```python
from build123d import *

# Parameters (mm, degrees)
SKETCH1_W           = 10
SKETCH1_H           = 10
BOSS_EXTRUDE1_DEPTH = 50
BOSS_EXTRUDE2_START = -45
SKETCH2_R           = 20
BOSS_EXTRUDE2_DEPTH = 2.5
FILLET2_R           = 2
FILLET3_R           = 5
FILLET4_R           = 5
SCALE1_SCALE        = 1.5


with BuildPart() as part:
    # Sketch1 → Boss-Extrude1 (new, symmetric)
    with BuildSketch(Plane(origin=(0, 0, 0), x_dir=(1, 0, 0), z_dir=(0, 1, 0))):
        Rectangle(SKETCH1_W, SKETCH1_H)
    extrude(amount=BOSS_EXTRUDE1_DEPTH, both=True)

    # Sketch2 → Boss-Extrude2 (add, symmetric)
    with BuildSketch(Plane(origin=(0, 50, 0), x_dir=(1, 0, 0), z_dir=(0, 1, 0)).offset(BOSS_EXTRUDE2_START)):
        with Locations(Location((0, 0, 0), (0, 0, 270))):
            Circle(SKETCH2_R)
    extrude(amount=BOSS_EXTRUDE2_DEPTH, both=True)

    # Fillet2
    fillet2_edges = [part.edges().sort_by_distance(p)[0] for p in [
        (5, -23.75, 5),
        (-5, -23.75, 5),
        (-5, -23.75, -5),
        (5, -23.75, -5),
    ]]
    fillet(fillet2_edges, radius=FILLET2_R)

    # Fillet3
    fillet3_edges = [part.edges().sort_by_distance(p)[0] for p in [
        (-5, 28.75, -5),
        (-5, 28.75, 5),
        (5, 28.75, 5),
        (5, 28.75, -5),
    ]]
    fillet(fillet3_edges, radius=FILLET3_R - 0.0001)  # a hair under: the kernel refuses the full size

    # Fillet4
    fillet4_edges = [part.edges().sort_by_distance(p)[0] for p in [
        (3.535563195, 50, -3.535563195),
        (3.535563195, 50, 3.535563195),
        (-3.535563195, 50, 3.535563195),
        (-3.535563195, 50, -3.535563195),
    ]]
    fillet(fillet4_edges, radius=FILLET4_R - 0.0001)  # a hair under: the kernel refuses the full size


with BuildPart() as part_1:
    # Scale1: scaled about (0, 0.040894901, 0)
    add(part.part.scale(SCALE1_SCALE).moved(Location((0, -0.02044745, 0))))


solid = part_1.part
```
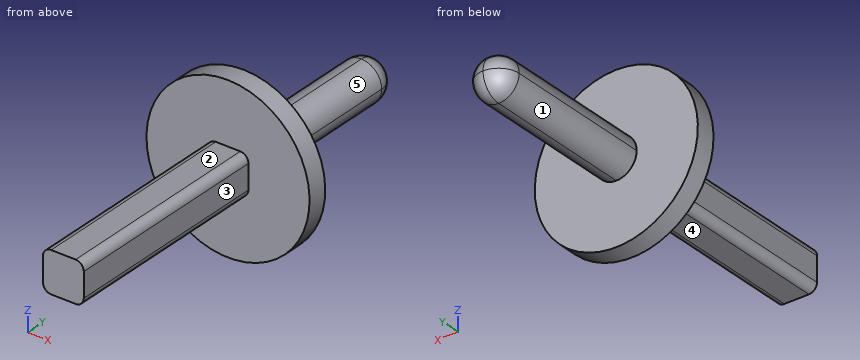
Geometry check sheet. Reference: the model listing, model coordinates, mm. Face numbers are marked on the shaded views. A direction names the side the tool comes from. Round coordinates to 2 decimals unless told otherwise and drop trailing zeros. Order: outer loops, then holes, each group sorted by start corner. A loop starts at its lowest first (then second) coordinate and runs counter-clockwise, first axis right, second up. Notation, with made-up numbers: M 5.25,-1.75 L 33.25,-1.75 A24 ccw 33.25,29.25 Z; hole C 69.25,-22.5 d8. An arc over 180 degrees is marked long. Write item = value, one per line.
Q1. Depth check by flat-ended pin: pin 1 Ø6 at (x, z) = (-16.5, -21.5) entering from -Y; pin 2 Ø10 at (y, z) = (-24, 2) entering from -X; pin 3 Ø7 at (x, y) = (1.5, -31) entering from +Z; pin 4 Ø1 at (y, z) = (-31, 9) entering from -X. Enter the tip coordinate at first touch or a pass-through.
Answer block:
pin_1 = 3.73
pin_2 = -7.5
pin_3 = 7.5
pin_4 = through
Q2. Scan lines: line 1 (Y direction, x = 14.5, z = -25); line 2 (Y direction, x = -4.5, z = -6.5); line 3 (Z direction, x = 19, y = 10). Record each from-to range of solid material in increasing order.
Answer block:
line_1 = 3.73 to 11.23
line_2 = -75.02 to 11.23
line_3 = -23.22 to 23.22
Q3. Section check D-D (x = 9). Enter the section's corners in (y, z).
Answer block:
outline = M 3.73,-28.62 L 11.23,-28.62 L 11.23,28.62 L 3.73,28.62 Z
Q4. Section check C-C (y = -13.5). Enter the section's corners in (x, z).
Answer block:
outline = M -7.5,-4.5 A3 ccw -4.5,-7.5 L 4.5,-7.5 A3 ccw 7.5,-4.5 L 7.5,4.5 A3 ccw 4.5,7.5 L -4.5,7.5 A3 ccw -7.5,4.5 Z
Q5. Set-up check for the marked faces 1, 2, 3, 4 and 5: record each of +Z, -Z, +X, -X, +Y, -Y from which the full face is reachable in a straight line by a thin tool's end or side.
Answer block:
face_1 = -Z, -X, +Y
face_2 = +Z, +X, -X, -Y
face_3 = +Z, -Z, +X, -Y
face_4 = -Z, +X, -X, -Y
face_5 = +Z, +X, +Y
Q6. Section check B-B (x = -24). Enter the section's corners in (y, z), plus the area to 3 significant figures.
Answer block:
outline = M 3.73,-18 L 11.23,-18 L 11.23,18 L 3.73,18 Z
area = 270 mm^2
